Autodesk Inventor part; units mm, degrees
ref_plane "Work Plane3" through (61.2399, 0, 54.5647) normal (0.6088, 0, -0.7933) x (-0.7933, 0, -0.6088)
ref_plane "YZ Plane" through (0, 0, 0) normal (1, 0, 0) x (0, 1, 0)
ref_plane "XZ Plane" through (0, 0, 0) normal (0, 1, 0) x (-1, 0, 0)
sketch "Sketch1" plane through (0, 0, 0) normal (0, 1, 0) x (-1, 0, 0)
  line L0 (0, 0) -> (48.2762, -0.0067)
  line L1 (-64.893, 49.805) -> (0, 0)
  line L2 (-40.6563, 51.3726) -> (-58.6663, 59.989)
  line L3 (-12.8113, 30.0018) -> (-40.6563, 51.3726)
  line L4 (48.2788, 29.9933) -> (-12.8113, 30.0018)
  arc A0 (-58.6663, 59.989) -> (-64.893, 49.805) centre (-61.2549, 54.5762) ccw
  arc A1 (48.2762, -0.0067) -> (48.2788, 29.9933) centre (48.2762, 14.9933) ccw
  point P0 (0, 0)
  dimension "d0" = 0
  dimension "d1" = 0
  dimension "d2" = 15
  dimension "d3" = 48.2762
  dimension "d4" = 48.2762
  dimension "d5" = 61.0901
  dimension "d6" = 109.5311
  dimension "d7" = 6
  dimension "d8" = 168.062
  dimension "d9" = 30
  dimension "d10" = 16
  dimension "d11" = 18.01
extrude "Extrusion1" add sketch "Sketch1" along normal blind 6
sketch "Sketch2" plane through (0, 6, 0) normal (0, 1, 0) x (1, 0, 0)
  arc A0 (-48.2762, 0.0067) -> (-48.2788, -29.9933) centre (-48.2762, -14.9933) ccw
  circle A1 centre (-48.2762, -14.9933) radius 15
  point P0 (0, 0)
  point P1 (-48.2788, -29.9933)
  point P2 (-48.2762, 0.0067)
extrude "Extrusion2" cut sketch "Sketch2" against normal blind 0.3
sketch "Sketch3" plane through (0, 6, 0) normal (0, 1, 0) x (1, 0, 0)
  circle A0 centre (-8.2762, -14.9988) radius 12
  arc A1 (-48.2762, 0.0067) -> (-48.2788, -29.9933) centre (-48.2762, -14.9933) ccw
  line L0 (-48.2788, -29.9933) -> (12.8113, -30.0018)
  point P0 (0, 0)
  point P1 (-63.2762, -14.992)
  dimension "d16" = 55
  dimension "d17" = 15
  dimension "d18" = 24
extrude "Extrusion3" cut sketch "Sketch3" against normal blind 10
sketch "Sketch8" plane through (0, 5.7, 0) normal (0, 1, 0) x (1, 0, 0)
  arc A0 (-48.2762, 0.0067) -> (-48.2788, -29.9933) centre (-48.2762, -14.9933) ccw
  circle A1 centre (-48.2762, -14.9933) radius 6.3
  point P0 (0, 0)
  dimension "d37" = 12.6
extrude "Extrusion4" cut sketch "Sketch8" against normal blind 10
chamfer "Chamfer1" distance 0.3 angle 45 1 edges at (-54.5762, 5.7, 14.9933) measured on face at (-46.8281, 5.7, 26.9329)
fillet "Fillet1" radius 15 1 edges at (0, 3, 0)
fillet "Fillet2" radius 5 1 edges at (12.8113, 3, 30.0018)
fillet "Fillet3" radius 10 1 edges at (40.6563, 3, 51.3726)
sketch "Sketch15" plane through (64.893, 0, 49.805) normal (0.6088, 0, -0.7933) x (-0.7933, 0, -0.6088)
  point P0 (81.8024, 0)
sketch "Sketch16" plane through (0, 6, 0) normal (0, 1, 0) x (1, 0, 0)
  point P0 (0, 0)
ref_plane "Work Plane3" through (61.2399, 0, 54.5647) normal (0.6088, 0, -0.7933) x (-0.7933, 0, -0.6088)
sketch "Sketch18" plane through (61.2399, 0, 54.5647) normal (0.6088, 0, -0.7933) x (-0.7933, 0, -0.6088)
  line L0 (0, 6) -> (76.7109, 6)
  line L1 (0, 6) -> (0, 3.5)
  line L2 (0, 0) -> (0, 6)
  line L3 (-2.5, 3.5) -> (-5, 6)
  line L4 (0, 6) -> (-6.0189, 6)
  line L5 (-2.5, 3.5) -> (0, 3.5)
  line L6 (-6.0189, 0) -> (-6.0189, 6)
  line L7 (-6.0189, 3) -> (0, 3) construction
  line L8 (0, 0) -> (0, 2.5)
  line L9 (-2.5, 2.5) -> (-5, 0)
  line L10 (-2.5, 2.5) -> (0, 2.5)
  line L11 (-5, 0) -> (0, 0)
  line L12 (17.2493, 0) -> (-1.2609, 0)
  point P0 (81.8024, 0)
  point P1 (-1.2609, 6)
  point P2 (0, 2.5)
  dimension "d75" = 2.5
  dimension "d76" = 2.5
  dimension "d77" = 5
revolve "Revolution1" cut sketch "Sketch18" angle 360 about axis through (61.2399, 6, 54.5647) along (0, -1, 0)
sketch "Sketch19" plane through (61.2399, 3.5, 54.5647) normal (0, 1, 0) x (1, 0, 0)
  circle A0 centre (0, 0) radius 2.5
  point P0 (-61.2399, 54.5647)
extrude "Extrusion6" cut sketch "Sketch19" against normal blind 10
properties part number "31-10-201-novi"
Model file for the job. Use its own axes, mm. A direction names the side the tool comes from. Round coordinates to 2 decimals unless told otherwise and drop trailing zeros. Order: outer loops, then holes, each group sorted by start corner. A loop starts at its lowest first (then second) coordinate and runs counter-clockwise, first axis right, second up.
(1) 3-axis set-ups, long thin cutter, end or side, ignore diameter. For faces 4 (the face through (-42, 5.7, 18)), 5 (the face through (2.3, 0, 21.5)): which of +Z, -Z, +X, -X, +Y, -Y reach the whole face in a straight line?
(2) Band-saw the part on D-D (z = 28.5). List the corners of the cut face in (x, y), then the cut area to 3 significant figures.
(3) Drill centre lines: line 1 (X direction, y = 4.75, z = 12); line 2 (Z direction, x = -32, y = 1.5); line 3 (Z direction, x = -2, y = 3.75). Where is each one in solid material? Low to high.
(4) Pull direction Z, two halves, no side cores. Call faces 1 (the face through (26.813, 2.958, 40.748)), 2 (the face through (-0.205, 3.042, 0.818)), 3 (the face through (63.74, 3.66, 55.47)): released by +Z, released by -Z, zero draft, split by the parting line, or undercut.
(5) Pin check, flat tips, straight feed: pin 1 (1 mm diameter, centred on x = -25.5, z = 15.5, fed in from -Y); pin 2 (1.5 mm diameter, centred on y = 3, z = 12, fed in from -X); pin 3 (3 mm diameter, centred on x = -12.5, y = 3.5, fed in from -Z); pin 4 (8 mm diameter, centred on x = 61.24, z = 54.56, fed in from +Y). Stop position of each tip, or through.
(6) Band-saw the part on B-B (z = 5). List the corners of the cut face in (x, y), then the cut area to 3 significant figures.
(7) Band-saw the part on A-A (x = -11). List the corners of the cut face in (y, z).
Verdict:
1. face 4: -X, +Y
1. face 5: +Z, -Z, +X, -X, -Y
2. outline: (-54.8, 0) - (37.13, 0) - (37.13, 6) - (-41.75, 6) - (-41.75, 5.7) - (-54.8, 5.7) - close
2. area: 548 mm2
3. line 1: x = -62.97 to -53.82, -42.73 to -19.9, 3.34 to 15.64
3. line 2: z = 0 to 30
3. line 3: z = 0.32 to 4.77, 25.23 to 30
4. face 1: released by +Z
4. face 2: released by -Z
4. face 3: undercut
5. pin 1: stops at y = 0
5. pin 2: stops at x = -63.11
5. pin 3: stops at z = 0
5. pin 4: stops at y = 5
6. outline: (-59.46, 0) - (-14.91, 0) - (-14.91, 6) - (-37.09, 6) - (-37.09, 5.7) - (-59.46, 5.7) - close; (-1.64, 0) - (6.51, 0) - (6.51, 6) - (-1.64, 6) - close
6. area: 310 mm2
7. outline: (0, 0) - (6, 0) - (6, 3.31) - (0, 3.31) - close; (0, 26.69) - (6, 26.69) - (6, 30) - (0, 30) - close
